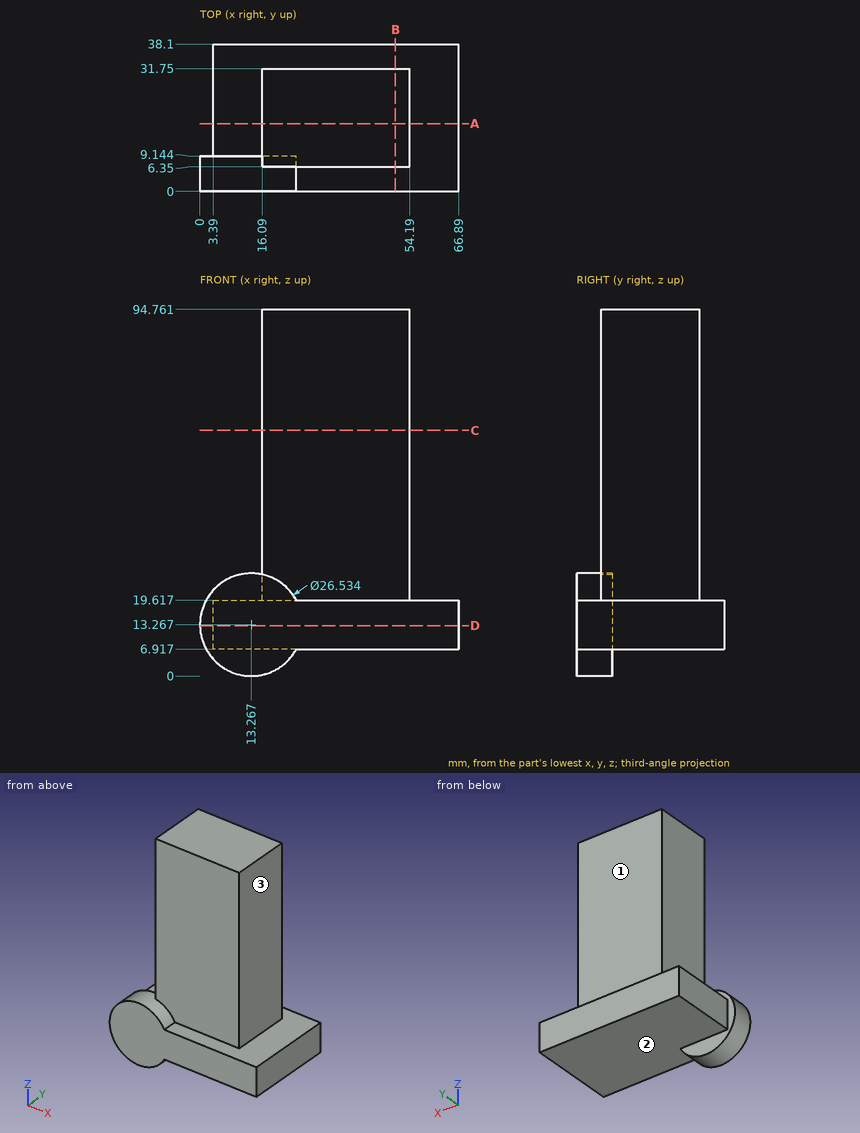
Geometry check sheet. Reference: drawing and pictorial views, mm from the part's lowest x, y, z. A direction names the side the tool comes from. Coordinates: 2 decimals unless noted, no trailing zeros. Order: outer loops, then holes, each group sorted by start corner. A loop starts at its lowest first (then second) coordinate and runs counter-clockwise, first axis right, second up. Notation, with made-up numbers: (73, -15) -> (82, -15) arc R16 cw to (82, 13) -> close; hole circle Ø11 at (30, -11.75). An arc over 180 degrees is marked (long way). Put each result on its own line as item: value. Start each with the question number.
1) Go/stop test with flat-tipped pins: pin 1 (2 mm diameter, centred on x = 52.5, y = 12, fed in from -Z); pin 2 (12 mm diameter, centred on x = 15, y = 5, fed in from -Z); pin 3 (10 mm diameter, centred on y = 25.5, z = 14.5, fed in from -X); pin 4 (11.5 mm diameter, centred on x = 31.5, z = 55.5, fed in from -Y). Record where each tip stops, or that it passes through.
2) Cross-section at A-A (y = 17.5). Enter the section's corners in (x, z), plus the area to 3 significant figures.
3) Tool access check on the marked faces 1, 2 and 3. Record the directions out of +Z, -Z, +X, -X, +Y, -Y that give a thin tool (end or side, any length) a straight path to the whole face; none if there is none.
4) Cross-section at B-B (x = 50.5). Enter the section's corners in (y, z), plus the area to 3 significant figures.
5) Material ranges on L1, parallel to Y at x = 47, z = 59.5; L2, parallel to Z at x = 60.5, y = 34.5; L3, parallel to Z at x = 44, y = 15, recorded low to high.
6) Cross-section at C-C (z = 63.5). Enter the section's corners in (x, y), plus the area to 3 significant figures.
7) Cross-section at D-D (z = 13). Enter the section's corners in (x, y), plus the area to 3 significant figures.
Geometry check:
1. pin 1: stops at z = 6.92
1. pin 2: stops at z = 0
1. pin 3: stops at x = 3.39
1. pin 4: stops at y = 6.35
2. outline: (3.39, 6.92) -> (66.89, 6.92) -> (66.89, 19.62) -> (54.19, 19.62) -> (54.19, 94.76) -> (16.09, 94.76) -> (16.09, 19.62) -> (3.39, 19.62) -> close
2. area: 3,670 mm^2
3. face 1: +Z, +X, -X, +Y
3. face 2: -Z, +X, +Y
3. face 3: +Z, +X, +Y, -Y
4. outline: (0, 6.92) -> (38.1, 6.92) -> (38.1, 19.62) -> (31.75, 19.62) -> (31.75, 94.76) -> (6.35, 94.76) -> (6.35, 19.62) -> (0, 19.62) -> close
4. area: 2,390 mm^2
5. L1: y = 6.35 to 31.75
5. L2: z = 6.92 to 19.62
5. L3: z = 6.92 to 94.76
6. outline: (16.09, 6.35) -> (54.19, 6.35) -> (54.19, 31.75) -> (16.09, 31.75) -> close
6. area: 968 mm^2
7. outline: (0, 0) -> (66.89, 0) -> (66.89, 38.1) -> (3.39, 38.1) -> (3.39, 9.14) -> (0, 9.14) -> close
7. area: 2,450 mm^2
